The drawing under review shows one solid part. Ordinate dimensions are in mm from its lowest x, y, z. A direction names the side the tool comes from. Give positions to 0.01 mm unless a question says otherwise; leave off trailing zeros. Order: outer loops, then holes, each group sorted by start corner. A loop starts at its lowest first (then second) coordinate and runs counter-clockwise, first axis right, second up. Notation, with made-up numbers: (55, 62.25) -> (110, 62.25) arc R16 ccw to (110, 83.25) -> close; hole circle Ø9 at (60, 43.25). An arc over 180 degrees is marked (long way). One line per item, written item: value. Start each with the question number.
1) The part is to be moulded in two halves that separate along X. For the marked faces 3, 4 and 5, say which applies: released by +X, released by -X, zero draft, split by the parting line, or undercut.
2) Consider section A-A (y = 36.5). State how many separate pieces and enclosed holes the cut face has, plus the area to 3 significant figures.
3) Consider section C-C (x = 27.5). State the section outline as (y, z) points.
4) Consider section B-B (y = 20). State the section outline as (x, z) points (1 decimal).
5) For pin 1 (0.7 mm diameter, centred on x = 32, z = 11, fed in from -Y); pin 2 (7.5 mm diameter, centred on x = 21.5, z = 11.5, fed in from +Y), all flat-tipped, find the tip position at first contact; note any pin that passes through.
6) Tool access review of the marked faces 1 and 2: name each direction out of +Z, -Z, +X, -X, +Y, -Y from which nothing blocks a thin tool from reaching the whole face with its end or side.
7) Consider section D-D (y = 26). State the section outline as (x, z) points (1 decimal).
8) Wall thickness on line 1 along X through (y, z) = (18, 22.25) (1 decimal); line 2 along Y through (x, z) = (39, 9.75) (1 decimal): over which ranges is each line inside the solid? List them lowest first. Write a range as from..to.
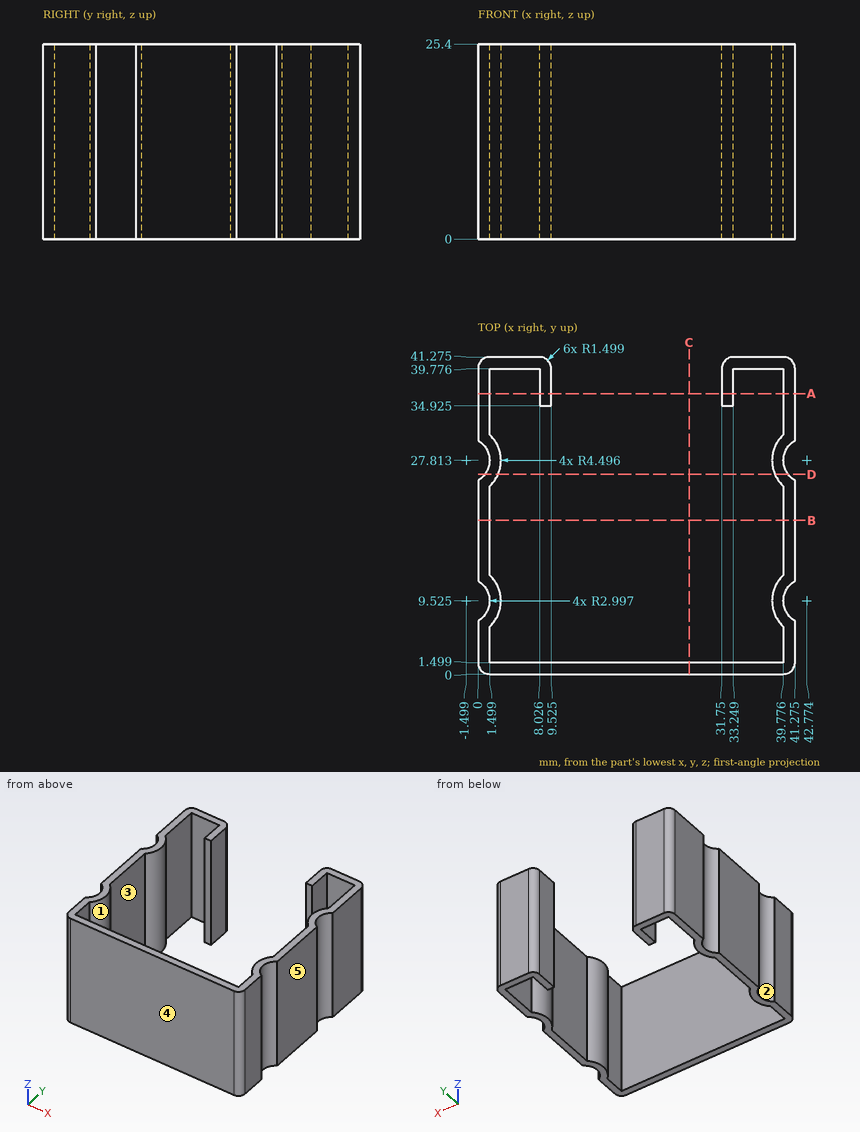
Checked values:
1. face 3: undercut
1. face 4: zero draft
1. face 5: released by +X
2. separate pieces: 4
2. enclosed holes: 0
2. area: 152 mm^2
3. outline: (0, 0) -> (1.5, 0) -> (1.5, 25.4) -> (0, 25.4) -> close
4. outline: (0, 0) -> (1.5, 0) -> (1.5, 25.4) -> (0, 25.4) -> close; (39.8, 0) -> (41.3, 0) -> (41.3, 25.4) -> (39.8, 25.4) -> close
5. pin 1: stops at y = 0
5. pin 2: stops at y = 1.5
6. face 1: +Z, -Z
6. face 2: +Z, -Z, -X
7. outline: (0.9, 0) -> (2.6, 0) -> (2.6, 25.4) -> (0.9, 25.4) -> close; (38.7, 0) -> (40.4, 0) -> (40.4, 25.4) -> (38.7, 25.4) -> close
8. line 1: x = 0..1.5, 39.8..41.3
8. line 2: y = 0..1.5, 7.1..12, 25.4..30.3, 39.8..41.3
